Study the drawing (mm; zero at the part's minimum x, y, z) and answer. Give positions to 0.01 mm unless a question says otherwise; leave off trailing zeros. Write each question's results on one line, items separated by ' | '. Start each with the question number.
1. Determine the mould class of the marked faces 1 and 2 for opening direction Y: released by +Y, released by -Y, zero draft, split by the parting line, or undercut.
2. Section B-B (y = 50.8) is taken. State how many separate pieces and enclosed holes the cut face has.
3. Find the intervals of material crossed by L1, parallel to X at y = 50.8, z = 0.75 (1 decimal); L2, parallel to Y at x = 69.85, z = 0.3 (1 decimal); L3, parallel to X at y = 12.5, z = 2.25 (1 decimal), in increasing order.
4. A flat-ended cylindrical pin translates along its axis: pin 1 (1 mm diameter, centred on x = 26.5, z = 3, fed in from -Y). Find the tip coordinate at first contact, or state that the pin passes through.
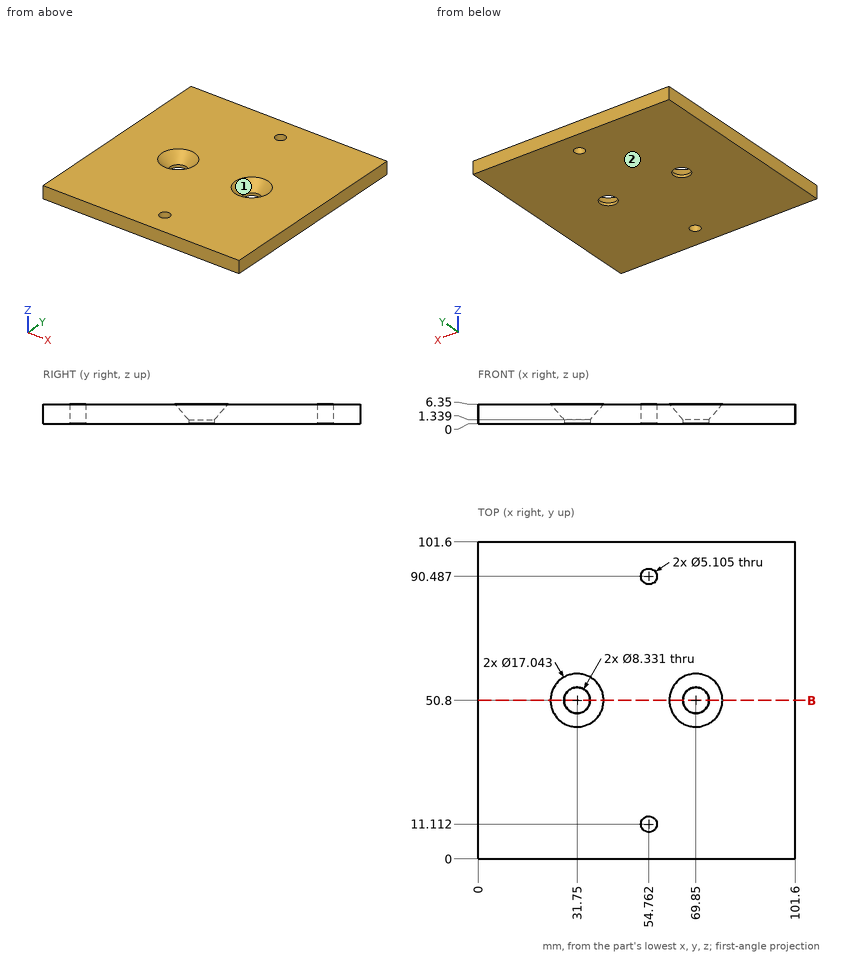
Reported:
1) face 1: undercut | face 2: zero draft
2) separate pieces: 3 | enclosed holes: 0
3) L1: 0 to 27.6, 35.9 to 65.7, 74 to 101.6 | L2: 0 to 46.6, 55 to 101.6 | L3: 0 to 52.6, 56.9 to 101.6
4) pin 1: y = 0
